Geometry: final body of the model. Coordinates: model frame, mm. Face numbers are marked on the shaded views. A direction names the side the tool comes from. Round coordinates to 2 decimals unless told otherwise and drop trailing zeros. Loops run counter-clockwise (first coordinate to the right, second up) from the corner with the lowest first, then second, coordinate; pieces in that order, holes last. Notation, with made-up numbers: (16, -3.5) - (32, -3.5) arc R25 ccw to (32, 15.5) - close; hole circle Ø11 at (19.25, 33.25). An arc over 180 degrees is marked (long way). Return JSON: item names as keys, results as strings. Group by question number.
1. Material intervals for probe 1 along Y at (x, z) = (5.25, 0); probe 2 along X at (y, z) = (34.5, -16); probe 3 along X at (y, z) = (9.5, 25.5), sorted ascending.
2. Section D-D on z = -50. Return loops of the section in (x, y), and give its area (3 significant figures).
3. Section C-C on x = 67. Return loops of the section in (y, z), and give its area (3 significant figures).
4. First-contact query: pin 1 Ø8 at (x, y) = (71.5, -27) entering from +Z; pin 2 Ø9 at (y, z) = (50.8, 0) entering from +X; pin 3 Ø10 at (y, z) = (-9, -36) entering from +X; pin 4 Ø1.8 at (x, z) = (54.5, 19.5) entering from +Y. Flat tips, straight axial feed; report the tip coordinate or a pass-through.
5. Section B-B on y = 50.8. Return loops of the section in (x, z), and give its area (3 significant figures).
6. Set-up query: the marked faces 4, 5, 6 and 7. Return all of +Z, -Z, +X, -X, +Y, -Y with unobstructed straight access to the full face (end or side cutting, diameter ignored); none if empty.
7. Draft query along X for the marked faces 1, 2 and 3. Return one class per face: +X half, -X half, draft (parallel to the pull), parting line (faces both ways), or undercut.
8. Section A-A on z = 0. Count the separate pieces of the cut face and the enclosed holes in it, and give its area (3 significant figures).
from build123d import *

# Parameters (mm, degrees)
SKETCH10_R           = 4
BOSS_EXTRUDE12_DEPTH = 10
SKETCH11_R           = 35
BOSS_EXTRUDE13_DEPTH = 40.8
SKETCH12_R           = 4
BOSS_EXTRUDE14_DEPTH = 6
SKETCH13_R           = 19.993
BOSS_EXTRUDE15_DEPTH = 75
SKETCH16_R           = 39
BOSS_EXTRUDE16_DEPTH = 3.5
CHAMFER1_SIZE        = 1
SKETCH17_R           = 4.05
CUT_EXTRUDE1_DEPTH   = 131.8


with BuildPart() as part:
    # Sketch10 → Boss-Extrude12 (new body)
    with BuildSketch(Plane(origin=(0, 0, 0), x_dir=(0, 0, -1), z_dir=(1, 0, 0))):
        with BuildLine():
            Line((-55.858638544, -18.55), (-11.864548032, 57.65))
            ThreePointArc((-11.864548032, 57.65), (0, 64.5), (11.864548032, 57.65))
            Line((11.864548032, 57.65), (55.858638544, -18.55))
            ThreePointArc((55.858638544, -18.55), (55.858638544, -32.25), (43.994090512, -39.1))
            Line((43.994090512, -39.1), (-43.994090512, -39.1))
            ThreePointArc((-43.994090512, -39.1), (-55.858638544, -32.25), (-55.858638544, -18.55))
        make_face()
        with Locations((0, 50.8)):
            Circle(SKETCH10_R, mode=Mode.SUBTRACT)
        with Locations((43.994090512, -25.4)):
            Circle(SKETCH10_R, mode=Mode.SUBTRACT)
        with Locations((-43.994090512, -25.4)):
            Circle(SKETCH10_R, mode=Mode.SUBTRACT)
    extrude(amount=BOSS_EXTRUDE12_DEPTH)

    # Sketch11 → Boss-Extrude13 (add)
    with BuildSketch(Plane(origin=(10, 0, 0), x_dir=(0, 0, -1), z_dir=(1, 0, 0))):
        Circle(SKETCH11_R)
    extrude(amount=BOSS_EXTRUDE13_DEPTH)

    # Sketch12 → Boss-Extrude14 (add)
    with BuildSketch(Plane(origin=(50.8, 0, 0), x_dir=(0, 0, -1), z_dir=(1, 0, 0))):
        with BuildLine():
            Line((-43.994090512, 39.1), (43.994090512, 39.1))
            ThreePointArc((43.994090512, 39.1), (55.858638544, 32.25), (55.858638544, 18.55))
            Line((55.858638544, 18.55), (11.864548032, -57.65))
            ThreePointArc((11.864548032, -57.65), (0, -64.5), (-11.864548032, -57.65))
            Line((-11.864548032, -57.65), (-55.858638544, 18.55))
            ThreePointArc((-55.858638544, 18.55), (-55.858638544, 32.25), (-43.994090512, 39.1))
        make_face()
        with Locations((43.994090512, 25.4)):
            Circle(SKETCH12_R, mode=Mode.SUBTRACT)
        with Locations((0, -50.8)):
            Circle(SKETCH12_R, mode=Mode.SUBTRACT)
        with Locations((-43.994090512, 25.4)):
            Circle(SKETCH12_R, mode=Mode.SUBTRACT)
    extrude(amount=BOSS_EXTRUDE14_DEPTH)

    # Sketch13 → Boss-Extrude15 (add)
    with BuildSketch(Plane(origin=(56.8, 0, 0), x_dir=(0, 0, -1), z_dir=(1, 0, 0))):
        Circle(SKETCH13_R)
    extrude(amount=BOSS_EXTRUDE15_DEPTH)

    # Sketch16 → Boss-Extrude16 (add)
    with BuildSketch(Plane(origin=(56.8, 0, 0), x_dir=(0, 0, -1), z_dir=(1, 0, 0))):
        Circle(SKETCH16_R)
    extrude(amount=BOSS_EXTRUDE16_DEPTH)

    # Chamfer1
    chamfer1_edges = [part.edges().sort_by_distance(p)[0] for p in [
        (131.8, 0, 19.993),
    ]]
    chamfer(chamfer1_edges, length=CHAMFER1_SIZE)

    # Sketch17 → Cut-Extrude1 (cut)
    with BuildSketch(Plane(origin=(131.8, 0, 0), x_dir=(0, 0, -1), z_dir=(1, 0, 0))):
        Circle(SKETCH17_R)
    extrude(amount=-CUT_EXTRUDE1_DEPTH, mode=Mode.SUBTRACT)


solid = part.part
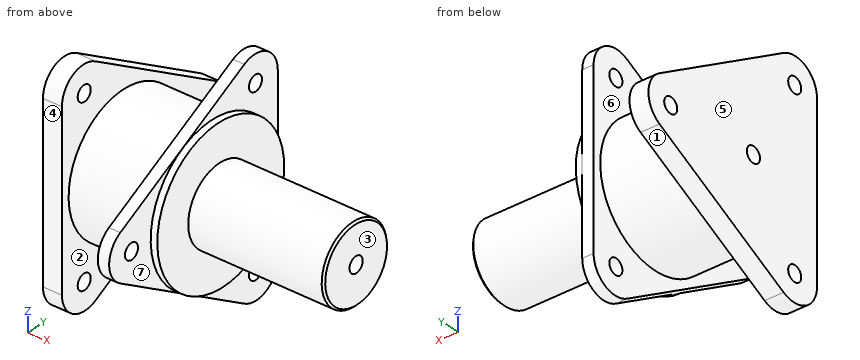
Taken from the geometry:
{
 "1": {"probe 1": "-39.1 to -4.05, 4.05 to 46.8, 54.8 to 64.5", "probe 2": "0 to 10, 50.8 to 60.3", "probe 3": "0 to 60.3"},
 "2": {"outline": "(0, -37.71) - (10, -37.71) - (10, -8.4) - (0, -8.4) - close; (50.8, 8.4) - (56.8, 8.4) - (56.8, 37.71) - (50.8, 37.71) - close", "area": "469 mm2"},
 "3": {"outline": "circle Ø39.99 at (0, 0); hole circle Ø8.1 at (0, 0)", "area": "1,200 mm2"},
 "4": {"pin 1": "through", "pin 2": "x = 10", "pin 3": "x = 60.3", "pin 4": "y = 39.1"},
 "5": {"outline": "(0, -15.82) - (10, -15.82) - (10, -4) - (0, -4) - close; (0, 4) - (10, 4) - (10, 15.82) - (0, 15.82) - close", "area": "236 mm2"},
 "6": {"face 4": "+Z, -Z, -X, -Y", "face 5": "+Z, -Z, -X, +Y, -Y", "face 6": "none", "face 7": "+X"},
 "7": {"face 1": "draft", "face 2": "undercut", "face 3": "+X half"},
 "8": {"separate pieces": "4", "enclosed holes": "0", "area": "6,450 mm2"}
}
